from build123d import *

# Parameters (mm, degrees)
F0_R     = 12.5
F1_DEPTH = 25
F0_R_2   = 10


with BuildPart() as f1:
    # F0 (on Front) → F1 (new body)
    with BuildSketch(Plane.XZ):
        Circle(F0_R)
    extrude(amount=F1_DEPTH)


with BuildPart() as f1b:
    # F0 (on Front) → F1, piece 2 (new body)
    with BuildSketch(Plane.XZ):
        with Locations((0, 40)):
            Circle(F0_R_2)
    extrude(amount=F1_DEPTH)


solid = f1.part
Build history of the part. All positions in model axes, mm. Coordinates: 2 decimals unless noted, no trailing zeros. Order: outer loops, then holes, each group sorted by start corner. A loop starts at its lowest first (then second) coordinate and runs counter-clockwise, first axis right, second up. Notation, with made-up numbers: (29.25, 83) -> (58.25, 83) arc R25 ccw to (58.25, 121) -> close; hole circle Ø4 at (35.5, 61.25). An arc over 180 degrees is marked (long way). One line per item, written item: value.
(1) Drop flat-ended pins along their axis: pin 1 Ø12 at (x, y) = (9, -12) entering from -Z; pin 2 Ø1 at (x, y) = (-3, -15) entering from -Z; pin 3 Ø2 at (y, z) = (-10.5, -8) entering from +X. Give the stop position or say it passes through.
Checked values:
pin 1: z = -12.13
pin 2: z = -12.25
pin 3: x = 10.36
(2) Probe line 1 (X direction, y = -2, z = 10.75); line 2 (Z direction, x = -1.5, y = -14); line 3 (Z direction, x = 3.5, y = -14.25). List the from-to ranges inside material, lowest first. Write a range as [from, to].
Checked values:
line 1: [-6.38, 6.38]
line 2: [-12.41, 12.41]
line 3: [-12, 12]
(3) Slice it at B-B, the plane y = -3.25. List the corners of the cut face in (x, z), plus the area to 3 significant figures.
Checked values:
outline: circle Ø25 at (0, 0)
area: 491 mm2
(4) Slice it at C-C, the plane x = -8.5. List the corners of the cut face in (y, z).
Checked values:
outline: (-25, -9.17) -> (0, -9.17) -> (0, 9.17) -> (-25, 9.17) -> close
(5) Slice it at A-A, the plane z = -2.75. List the corners of the cut face in (x, y), plus the area to 3 significant figures.
Checked values:
outline: (-12.19, -25) -> (12.19, -25) -> (12.19, 0) -> (-12.19, 0) -> close
area: 610 mm2
